For this review, take the finished solid that the model builds, in its own axes (mm). Coordinates: 2 decimals unless noted, no trailing zeros. Loops run counter-clockwise (first coordinate to the right, second up) from the corner with the lowest first, then second, coordinate; pieces in that order, holes last. Notation, with made-up numbers: M 1,-8.75 L 35,-8.75 A23 ccw 35,1.25 Z; hole C -24.5,-16 d3. An arc over 180 degrees is marked long. Write item = value, one per line.
from build123d import *

# Parameters (mm, degrees)
F0_R     = 2
F1_DEPTH = 50


with BuildPart() as f1:
    # F0 (on Top) → F1 (new body)
    with BuildSketch(Plane.XY):
        with BuildLine():
            ThreePointArc((-6.9790131878, 1.9979447669), (-5.7, 0), (-6.9790131878, -1.9979447669))
            add(Edge.make_bspline(
                [(-6.9790131878, -1.9979447669), (0, -6.1313006259), (6.9790131878, -1.9979447669)],
                knots=[0.6075302167, 0.6075302167, 0.6075302167, 2.5340624369, 2.5340624369, 2.5340624369], degree=2, weights=[1, 0.570841362, 1]))
            ThreePointArc((6.9790131878, -1.9979447669), (5.7, 0), (6.9790131878, 1.9979447669))
            add(Edge.make_bspline(
                [(6.9790131878, 1.9979447669), (0, 6.1313006259), (-6.9790131878, 1.9979447669)],
                knots=[3.7491228703, 3.7491228703, 3.7491228703, 5.6756550905, 5.6756550905, 5.6756550905], degree=2, weights=[1, 0.570841362, 1]))
        make_face()
        Circle(F0_R, mode=Mode.SUBTRACT)
    extrude(amount=F1_DEPTH)


solid = f1.part
Q1. For line 1 along Y through (x, z) = (0, 28.5); line 2 along Y through (x, z) = (-1.75, 15); line 3 along X through (y, z) = (0.75, 41), list the stretches that pass through material, from the lowest coordinate up.
Solved:
line_1 = -3.5 to -2, 2 to 3.5
line_2 = -3.43 to -0.97, 0.97 to 3.43
line_3 = -5.83 to -1.85, 1.85 to 5.83
Q2. For pin 1 Ø3 at (x, z) = (3, 25) entering from -Y; pin 2 Ø5 at (x, z) = (5, 13) entering from -Y; pin 3 Ø1 at (x, z) = (-1, 10.5) entering from -Y; pin 4 Ø2.5 at (x, y) = (0, 0) entering from +Z (3 decimals), all flat-tipped, find the tip position at first contact; note any pin that passes through.
Solved:
pin_1 = -3.45
pin_2 = -3.35
pin_3 = -3.49
pin_4 = through
Q3. Add section A-A (y = 0). Write out the cut boundary in (x, z).
Solved:
outline = M -5.7,0 L -2,0 L -2,50 L -5.7,50 Z; M 2,0 L 5.7,0 L 5.7,50 L 2,50 Z
Q4. Draft analysis for pull direction Y (two halves, no side actions). For faces 1 (the face through (0, -2, 25)), 2 (the face through (-2, 1, 0)), state which applies: +Y half, -Y half, draft (parallel to the pull), parting line (faces both ways), or undercut.
Solved:
face_1 = undercut
face_2 = draft
